from build123d import *

# Parameters (mm, degrees)
SKETCH1_W           = 203.2
SKETCH1_H           = 101.6
SKETCH1_R           = 1.6
SKETCH1_W_2         = 68.58
SKETCH1_H_2         = 54.953705786
BOSS_EXTRUDE1_DEPTH = 3.175
SKETCH2_R           = 1.6
CUT_EXTRUDE1_DEPTH  = 10


with BuildPart() as part:
    # Sketch1 → Boss-Extrude1 (new body)
    with BuildSketch(Plane(origin=(0, 0, 0), x_dir=(1, 0, 0), z_dir=(0, 1, 0))):
        with Locations((101.6, -50.8)):
            Rectangle(SKETCH1_W, SKETCH1_H)
        with Locations(Location((20.431013284, -94.769213223, 0), (0, 0, 270))):
            Circle(SKETCH1_R, mode=Mode.SUBTRACT)
        with Locations(Location((20.431013284, -81.10763967, 0), (0, 0, 270))):
            Circle(SKETCH1_R, mode=Mode.SUBTRACT)
        Polygon((81.28, -23.323147107), (81.28, -78.276852893), (12.405089541, -78.276852893), (12.405089541, -74.276852893), (12.7, -74.276852893), (12.7, -27.323147107), (12.648382796, -27.323147107), (12.648382796, -23.323147107), align=None, mode=Mode.SUBTRACT)
        with Locations(Location((85, -63.98136033, 0), (0, 0, 270))):
            Circle(SKETCH1_R, mode=Mode.SUBTRACT)
        with Locations(Location((85.6, -51.6, 0), (0, 0, 270))):
            Circle(SKETCH1_R, mode=Mode.SUBTRACT)
        with Locations(Location((182.768986716, -94.769213223, 0), (0, 0, 270))):
            Circle(SKETCH1_R, mode=Mode.SUBTRACT)
        with Locations(Location((182.768986716, -81.10763967, 0), (0, 0, 270))):
            Circle(SKETCH1_R, mode=Mode.SUBTRACT)
        with Locations(Location((118.2, -63.98136033, 0), (0, 0, 270))):
            Circle(SKETCH1_R, mode=Mode.SUBTRACT)
        with Locations(Location((117.6, -51.6, 0), (0, 0, 270))):
            Circle(SKETCH1_R, mode=Mode.SUBTRACT)
        with Locations((156.21, -50.8)):
            Rectangle(SKETCH1_W_2, SKETCH1_H_2, mode=Mode.SUBTRACT)
        with Locations(Location((85.6, -41.6, 0), (0, 0, 270))):
            Circle(SKETCH1_R, mode=Mode.SUBTRACT)
        with Locations(Location((85.6, -31.6, 0), (0, 0, 270))):
            Circle(SKETCH1_R, mode=Mode.SUBTRACT)
        with Locations(Location((20.431013284, -20.49236033, 0), (0, 0, 270))):
            Circle(SKETCH1_R, mode=Mode.SUBTRACT)
        with Locations(Location((20.431013284, -6.830786777, 0), (0, 0, 270))):
            Circle(SKETCH1_R, mode=Mode.SUBTRACT)
        with Locations(Location((85, -20.49236033, 0), (0, 0, 270))):
            Circle(SKETCH1_R, mode=Mode.SUBTRACT)
        with Locations(Location((85, -6.830786777, 0), (0, 0, 270))):
            Circle(SKETCH1_R, mode=Mode.SUBTRACT)
        with Locations(Location((117.6, -41.6, 0), (0, 0, 270))):
            Circle(SKETCH1_R, mode=Mode.SUBTRACT)
        with Locations(Location((117.6, -31.6, 0), (0, 0, 270))):
            Circle(SKETCH1_R, mode=Mode.SUBTRACT)
        with Locations(Location((118.2, -20.49236033, 0), (0, 0, 270))):
            Circle(SKETCH1_R, mode=Mode.SUBTRACT)
        with Locations(Location((118.2, -6.830786777, 0), (0, 0, 270))):
            Circle(SKETCH1_R, mode=Mode.SUBTRACT)
        with Locations(Location((182.768986716, -20.49236033, 0), (0, 0, 270))):
            Circle(SKETCH1_R, mode=Mode.SUBTRACT)
        with Locations(Location((182.768986716, -6.830786777, 0), (0, 0, 270))):
            Circle(SKETCH1_R, mode=Mode.SUBTRACT)
    extrude(amount=-BOSS_EXTRUDE1_DEPTH)

    # Sketch2 → Cut-Extrude1 (cut)
    with BuildSketch(Plane.XZ.offset(3.175)):
        with Locations(Location((6.35, 12.7, 0), (0, 0, 270))):
            Circle(SKETCH2_R)
        with Locations(Location((6.35, 95.25, 0), (0, 0, 270))):
            Circle(SKETCH2_R)
        with Locations(Location((6.35, 88.9, 0), (0, 0, 270))):
            Circle(SKETCH2_R)
        with Locations(Location((196.85, 6.35, 0), (0, 0, 270))):
            Circle(SKETCH2_R)
        with Locations(Location((196.85, 12.7, 0), (0, 0, 270))):
            Circle(SKETCH2_R)
        with Locations(Location((196.85, 88.9, 0), (0, 0, 270))):
            Circle(SKETCH2_R)
        with Locations(Location((6.35, 6.35, 0), (0, 0, 270))):
            Circle(SKETCH2_R)
        with Locations(Location((196.85, 95.25, 0), (0, 0, 270))):
            Circle(SKETCH2_R)
    extrude(amount=-CUT_EXTRUDE1_DEPTH, mode=Mode.SUBTRACT)


solid = part.part
Read the model definition and answer for the solid it produces. Units are mm, in the model's axes. Round coordinates to 2 decimals unless told otherwise and drop trailing zeros. Write each loop counter-clockwise with the first axis right and the second up, starting at its lowest first coordinate (ties: lowest second). Pieces come first, ordered by that corner, then holes.
Q1. Find section B-B on z = 59. Determine the outline of the cut face in (x, y) (3 decimals).
Values:
outline: (0, -3.175) - (12.7, -3.175) - (12.7, 0) - (0, 0) - close; (81.28, -3.175) - (121.92, -3.175) - (121.92, 0) - (81.28, 0) - close; (190.5, -3.175) - (203.2, -3.175) - (203.2, 0) - (190.5, 0) - close
Q2. Find section C-C on y = -0.55. State how many separate pieces and enclosed holes the cut face has, and give its area (3 significant figures).
Values:
separate pieces: 1
enclosed holes: 30
area: 12,900 mm2
Q3. Straight lines are drawn through the part: line 1 (X direction, y = -2.85, z = 72); line 2 (X direction, y = -2.35, z = 94); line 3 (X direction, y = -1.9, z = 81.5). For each, find the intervals that lie inside material, in ascending order.
Values:
line 1: x = 0 to 12.7, 81.28 to 121.92, 190.5 to 203.2
line 2: x = 0 to 5.35, 7.35 to 19.03, 21.83 to 181.37, 184.17 to 195.85, 197.85 to 203.2
line 3: x = 0 to 18.88, 21.98 to 181.22, 184.32 to 203.2
Q4. Find section A-A on x = 149. Determine the outline of the cut face in (y, z) (3 decimals), and give its area (3 significant figures).
Values:
outline: (-3.175, 0) - (0, 0) - (0, 23.323) - (-3.175, 23.323) - close; (-3.175, 78.277) - (0, 78.277) - (0, 101.6) - (-3.175, 101.6) - close
area: 148 mm2
Q5. A flat-ended cylindrical pin translates along its axis: P1, Ø2.5, axis at x = 20.43, z = 20.49, coming from the +Y side. Find the tip coordinate at first contact, or state that the pin passes through.
Values:
P1: passes through
